Answer from the drawing. Dimensions are ordinates in mm from the lowest x, y and z of the part. Coordinates: 2 decimals unless noted, no trailing zeros. Write each loop counter-clockwise with the first axis right and the second up, starting at its lowest first coordinate (ties: lowest second). Pieces come first, ordered by that corner, then holes.
1) The part is cut by section A-A (y = 1.15). Determine the outline of the cut face in (x, z) (1 decimal), then the cut area to 3 significant figures.
2) Each of these flat-tipped pins is pushed along its axis until it touches: pin 1 Ø1 at (x, z) = (12.5, 2) entering from +Y (1 decimal); pin 2 Ø1 at (y, z) = (2.5, 6) entering from +X; pin 3 Ø5 at (x, z) = (2.54, 6.67) entering from -Y; pin 4 Ø2 at (x, y) = (1.5, 0.5) entering from -Z. Where does it stop, or does it pass through?
3) The part is cut by section C-C (z = 12). Determine the outline of the cut face in (x, y) (1 decimal), then the cut area to 3 significant figures.
4) The part is cut by section B-B (x = 2.54). Determine the outline of the cut face in (y, z) (1 decimal).
5) Find the intervals of material crossed by line 1 (X direction, y = 2.2, z = 8.5) (1 decimal); line 2 (X direction, y = 0.8, z = 7.75) (1 decimal); line 3 (Z direction, x = 2.54, y = 1.85) (1 decimal), in increasing order.
6) The part is cut by section D-D (x = 4.5). Determine the outline of the cut face in (y, z) (1 decimal).
7) Determine the mould class of the marked faces 1, 2, 3 and 4 for opening direction Z: +Z half, -Z half, draft (parallel to the pull), parting line (faces both ways), or undercut.
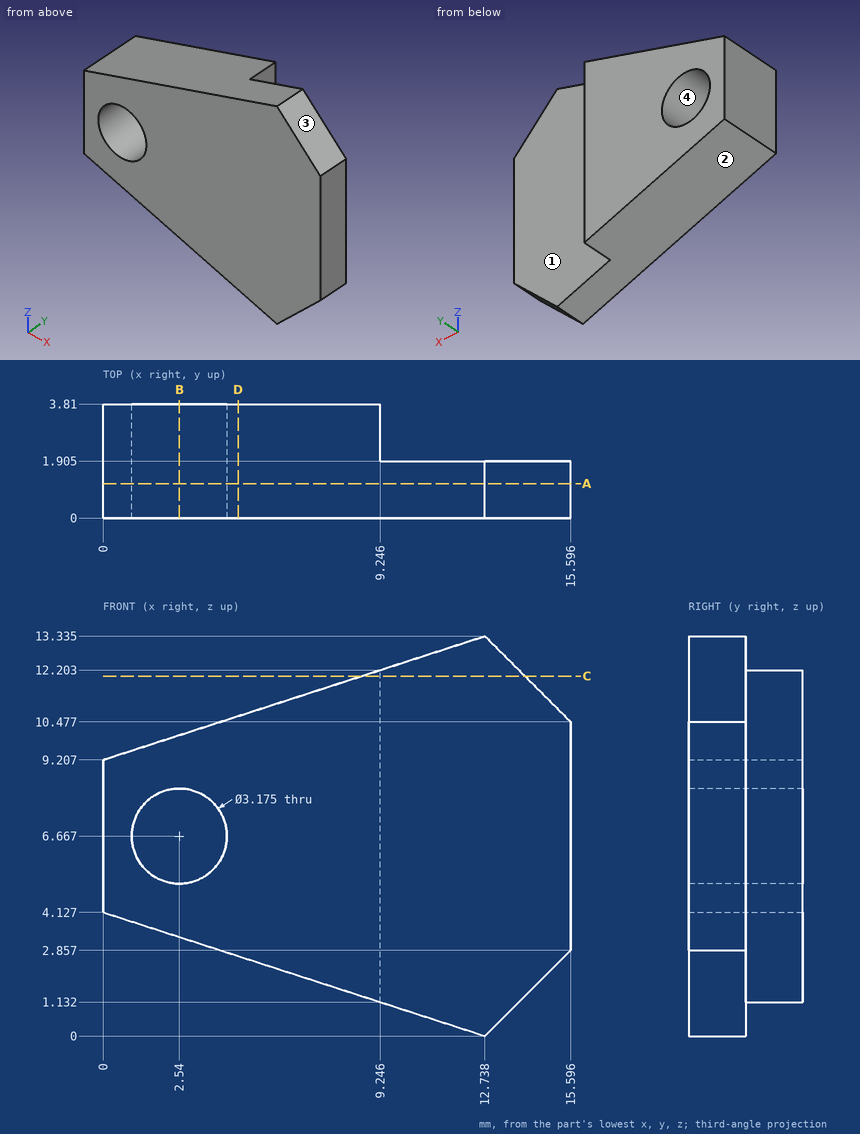
Reported:
1. outline: (0, 4.1) - (12.7, 0) - (15.6, 2.9) - (15.6, 10.5) - (12.7, 13.3) - (0, 9.2) - close; hole circle Ø3.2 at (2.5, 6.7)
1. area: 139 mm2
2. pin 1: stops at y = 1.9
2. pin 2: stops at x = 9.25
2. pin 3: stops at y = 0
2. pin 4: stops at z = 3.32
3. outline: (8.6, 0) - (14.1, 0) - (14.1, 1.9) - (9.2, 1.9) - (9.2, 3.8) - (8.6, 3.8) - close
3. area: 11.6 mm2
4. outline: (0, 3.3) - (3.8, 3.3) - (3.8, 5.1) - (0, 5.1) - close; (0, 8.3) - (3.8, 8.3) - (3.8, 10) - (0, 10) - close
5. line 1: x = 0 to 9.2
5. line 2: x = 0 to 1.4, 3.7 to 15.6
5. line 3: z = 3.3 to 5.1, 8.3 to 10
6. outline: (0, 2.7) - (3.8, 2.7) - (3.8, 10.7) - (0, 10.7) - close
7. face 1: draft
7. face 2: -Z half
7. face 3: +Z half
7. face 4: undercut
